CAD build for the part. Positions are in the model's coordinates, mm. A direction names the side the tool comes from. Round coordinates to 2 decimals unless told otherwise and drop trailing zeros. Write each loop counter-clockwise with the first axis right and the second up, starting at its lowest first coordinate (ties: lowest second). Pieces come first, ordered by that corner, then holes. Notation, with made-up numbers: (37.5, 69) -> (92.5, 69) arc R27 cw to (92.5, 105) -> close; hole circle Ø5 at (8.5, 34). An arc over 180 degrees is marked (long way). Answer in a Markdown table with one row per item. Add a question column.
```python
from build123d import *

# Parameters (mm, degrees)
BOSS_EXTRUDE1_DEPTH     = 56
CUT_EXTRUDE1_DEPTH      = 11
SKETCH6_R               = 11.25
SKETCH6_R_2             = 11
CUT_EXTRUDE3_DEPTH      = 7
CUT_EXTRUDE4_REACH      = 182.499
SKETCH7_R               = 1.55
SKETCH8_R               = 2.75
SKETCH8_R_2             = 1.55
CUT_EXTRUDE5_DEPTH      = 3
SKETCH9_R               = 4.5
SKETCH9_R_2             = 2.75
CUT_EXTRUDE6_DEPTH      = 5
CUT_EXTRUDE7_DEPTH      = 181.499307478
CUT_EXTRUDE7_DEPTH_BACK = 181.499307478
SKETCH9_3_R             = 2.75
FILLET1_R               = 10
FILLET2_R               = 25
FILLET3_R               = 5
FILLET4_R               = 2


with BuildPart() as part:
    # Sketch1 → Boss-Extrude1 (new, symmetric)
    with BuildSketch(Plane.XY):
        Polygon((130, 0), (130, 130), (112, 130), (112, 18), (0, 18), (0, 0), align=None)
    extrude(amount=BOSS_EXTRUDE1_DEPTH, both=True)

    # Sketch2 → Cut-Extrude1 (cut)
    with BuildSketch(Plane(origin=(130, 0, 0), x_dir=(0, 0, -1), z_dir=(1, 0, 0))):
        with BuildLine():
            Line((-20.060660172, 81.717766953), (-17.432233047, 79.089339828))
            ThreePointArc((-17.432233047, 79.089339828), (-16.945598024, 78.764180701), (-16.371572875, 78.65))
            Line((-16.371572875, 78.65), (16.371572875, 78.65))
            ThreePointArc((16.371572875, 78.65), (16.945598024, 78.764180701), (17.432233047, 79.089339828))
            Line((17.432233047, 79.089339828), (20.060660172, 81.717766953))
            ThreePointArc((20.060660172, 81.717766953), (20.385819299, 82.204401976), (20.5, 82.778427125))
            Line((20.5, 82.778427125), (20.5, 115.521572875))
            ThreePointArc((20.5, 115.521572875), (20.385819299, 116.095598024), (20.060660172, 116.582233047))
            Line((20.060660172, 116.582233047), (17.432233047, 119.210660172))
            ThreePointArc((17.432233047, 119.210660172), (16.945598024, 119.535819299), (16.371572875, 119.65))
            Line((16.371572875, 119.65), (-16.371572875, 119.65))
            ThreePointArc((-16.371572875, 119.65), (-16.945598024, 119.535819299), (-17.432233047, 119.210660172))
            Line((-17.432233047, 119.210660172), (-20.060660172, 116.582233047))
            ThreePointArc((-20.060660172, 116.582233047), (-20.385819299, 116.095598024), (-20.5, 115.521572875))
            Line((-20.5, 115.521572875), (-20.5, 82.778427125))
            ThreePointArc((-20.5, 82.778427125), (-20.385819299, 82.204401976), (-20.060660172, 81.717766953))
        make_face()
        with BuildLine():
            Line((-20.767766953, 81.010660172), (-18.139339828, 78.382233047))
            ThreePointArc((-18.139339828, 78.382233047), (-17.328281456, 77.840301169), (-16.371572875, 77.65))
            Line((-16.371572875, 77.65), (16.371572875, 77.65))
            ThreePointArc((16.371572875, 77.65), (17.328281456, 77.840301169), (18.139339828, 78.382233047))
            Line((18.139339828, 78.382233047), (20.767766953, 81.010660172))
            ThreePointArc((20.767766953, 81.010660172), (21.309698831, 81.821718544), (21.5, 82.778427125))
            Line((21.5, 82.778427125), (21.5, 115.521572875))
            ThreePointArc((21.5, 115.521572875), (21.309698831, 116.478281456), (20.767766953, 117.289339828))
            Line((20.767766953, 117.289339828), (18.139339828, 119.917766953))
            ThreePointArc((18.139339828, 119.917766953), (17.328281456, 120.459698831), (16.371572875, 120.65))
            Line((16.371572875, 120.65), (-16.371572875, 120.65))
            ThreePointArc((-16.371572875, 120.65), (-17.328281456, 120.459698831), (-18.139339828, 119.917766953))
            Line((-18.139339828, 119.917766953), (-20.767766953, 117.289339828))
            ThreePointArc((-20.767766953, 117.289339828), (-21.309698831, 116.478281456), (-21.5, 115.521572875))
            Line((-21.5, 115.521572875), (-21.5, 82.778427125))
            ThreePointArc((-21.5, 82.778427125), (-21.309698831, 81.821718544), (-20.767766953, 81.010660172))
        make_face()
    extrude(amount=-CUT_EXTRUDE1_DEPTH, mode=Mode.SUBTRACT)

    # Sketch6 → Cut-Extrude3 (cut)
    with BuildSketch(Plane.ZY.offset(-119)):
        with Locations(Location((0, 99.15, 0), (0, 0, 90))):
            Circle(SKETCH6_R)
        with Locations((0, 99.15)):
            Circle(SKETCH6_R_2, mode=Mode.SUBTRACT)
    extrude(amount=CUT_EXTRUDE3_DEPTH, mode=Mode.SUBTRACT)


with BuildPart() as cut_extrude3_kept_piece:
    # of the separate pieces the step leaves, the one the design keeps (cut_extrude3_pieces_kept)
    add(part.part.solids().sort_by_distance((130, 0, -56))[0])

    # Sketch7 → Cut-Extrude4 (cut, up to next)
    with BuildSketch(Plane.ZY.offset(-112), mode=Mode.PRIVATE) as cut_extrude4_sk1:
        with Locations(Location((-15.5, 83.65, 0), (0, 0, 270))):
            Circle(SKETCH7_R)
    cut_extrude4_tool1 = extrude(cut_extrude4_sk1.sketch, amount=-CUT_EXTRUDE4_REACH, mode=Mode.PRIVATE) & cut_extrude3_kept_piece.part
    # Sketch7 → Cut-Extrude4 (cut, up to next)
    with BuildSketch(Plane.ZY.offset(-112), mode=Mode.PRIVATE) as cut_extrude4_sk2:
        with Locations(Location((15.5, 83.65, 0), (0, 0, 270))):
            Circle(SKETCH7_R)
    cut_extrude4_tool2 = extrude(cut_extrude4_sk2.sketch, amount=-CUT_EXTRUDE4_REACH, mode=Mode.PRIVATE) & cut_extrude3_kept_piece.part
    # Sketch7 → Cut-Extrude4 (cut, up to next)
    with BuildSketch(Plane.ZY.offset(-112), mode=Mode.PRIVATE) as cut_extrude4_sk3:
        with Locations(Location((15.5, 114.65, 0), (0, 0, 270))):
            Circle(SKETCH7_R)
    cut_extrude4_tool3 = extrude(cut_extrude4_sk3.sketch, amount=-CUT_EXTRUDE4_REACH, mode=Mode.PRIVATE) & cut_extrude3_kept_piece.part
    # Sketch7 → Cut-Extrude4 (cut, up to next)
    with BuildSketch(Plane.ZY.offset(-112), mode=Mode.PRIVATE) as cut_extrude4_sk4:
        with Locations(Location((-15.5, 114.65, 0), (0, 0, 270))):
            Circle(SKETCH7_R)
    cut_extrude4_tool4 = extrude(cut_extrude4_sk4.sketch, amount=-CUT_EXTRUDE4_REACH, mode=Mode.PRIVATE) & cut_extrude3_kept_piece.part
    add(cut_extrude4_tool1.solids().sort_by_distance((112, 83.65, -15.5))[0], mode=Mode.SUBTRACT)
    add(cut_extrude4_tool2.solids().sort_by_distance((112, 83.65, 15.5))[0], mode=Mode.SUBTRACT)
    add(cut_extrude4_tool3.solids().sort_by_distance((112, 114.65, 15.5))[0], mode=Mode.SUBTRACT)
    add(cut_extrude4_tool4.solids().sort_by_distance((112, 114.65, -15.5))[0], mode=Mode.SUBTRACT)

    # Sketch8 → Cut-Extrude5 (cut)
    # profile 1 of 4: a face of its own
    with BuildSketch(Plane.ZY.offset(-112)):
        with Locations(Location((-15.5, 114.65, 0), (0, 0, 270))):
            Circle(SKETCH8_R)
        with Locations(Location((-15.5, 114.65, 0), (0, 0, 270))):
            Circle(SKETCH8_R_2, mode=Mode.SUBTRACT)
    # profile 2 of 4: a face of its own
    with BuildSketch(Plane.ZY.offset(-112)):
        with Locations(Location((15.5, 114.65, 0), (0, 0, 270))):
            Circle(SKETCH8_R)
        with Locations(Location((15.5, 114.65, 0), (0, 0, 270))):
            Circle(SKETCH8_R_2, mode=Mode.SUBTRACT)
    # profile 3 of 4: a face of its own
    with BuildSketch(Plane.ZY.offset(-112)):
        with Locations(Location((15.5, 83.65, 0), (0, 0, 270))):
            Circle(SKETCH8_R)
        with Locations(Location((15.5, 83.65, 0), (0, 0, 270))):
            Circle(SKETCH8_R_2, mode=Mode.SUBTRACT)
    # profile 4 of 4: a face of its own
    with BuildSketch(Plane.ZY.offset(-112)):
        with Locations(Location((-15.5, 83.65, 0), (0, 0, 270))):
            Circle(SKETCH8_R)
        with Locations(Location((-15.5, 83.65, 0), (0, 0, 270))):
            Circle(SKETCH8_R_2, mode=Mode.SUBTRACT)
    extrude(amount=-CUT_EXTRUDE5_DEPTH, mode=Mode.SUBTRACT)

    # Sketch9 → Cut-Extrude6 (cut)
    # profile 1 of 8: a face of its own
    with BuildSketch(Plane(origin=(0, 18, 0), x_dir=(1, 0, 0), z_dir=(0, 1, 0))):
        with Locations(Location((15, -41, 0), (0, 0, 180))):
            Circle(SKETCH9_R)
        with Locations((15, -41)):
            Circle(SKETCH9_R_2, mode=Mode.SUBTRACT)
    # profile 2 of 8: a face of its own
    with BuildSketch(Plane(origin=(0, 18, 0), x_dir=(1, 0, 0), z_dir=(0, 1, 0))):
        with Locations((15, -41)):
            Circle(SKETCH9_R_2)
    # profile 3 of 8: a face of its own
    with BuildSketch(Plane(origin=(0, 18, 0), x_dir=(1, 0, 0), z_dir=(0, 1, 0))):
        with Locations(Location((15, 41, 0), (0, 0, 180))):
            Circle(SKETCH9_R)
        with Locations((15, 41)):
            Circle(SKETCH9_R_2, mode=Mode.SUBTRACT)
    # profile 4 of 8: a face of its own
    with BuildSketch(Plane(origin=(0, 18, 0), x_dir=(1, 0, 0), z_dir=(0, 1, 0))):
        with Locations((15, 41)):
            Circle(SKETCH9_R_2)
    # profile 5 of 8: a face of its own
    with BuildSketch(Plane(origin=(0, 18, 0), x_dir=(1, 0, 0), z_dir=(0, 1, 0))):
        with Locations(Location((97, 41, 0), (0, 0, 180))):
            Circle(SKETCH9_R)
        with Locations((97, 41)):
            Circle(SKETCH9_R_2, mode=Mode.SUBTRACT)
    # profile 6 of 8: a face of its own
    with BuildSketch(Plane(origin=(0, 18, 0), x_dir=(1, 0, 0), z_dir=(0, 1, 0))):
        with Locations((97, 41)):
            Circle(SKETCH9_R_2)
    # profile 7 of 8: a face of its own
    with BuildSketch(Plane(origin=(0, 18, 0), x_dir=(1, 0, 0), z_dir=(0, 1, 0))):
        with Locations(Location((97, -41, 0), (0, 0, 180))):
            Circle(SKETCH9_R)
        with Locations((97, -41)):
            Circle(SKETCH9_R_2, mode=Mode.SUBTRACT)
    # profile 8 of 8: a face of its own
    with BuildSketch(Plane(origin=(0, 18, 0), x_dir=(1, 0, 0), z_dir=(0, 1, 0))):
        with Locations((97, -41)):
            Circle(SKETCH9_R_2)
    extrude(amount=-CUT_EXTRUDE6_DEPTH, mode=Mode.SUBTRACT)

    # Sketch9<3> → Cut-Extrude7 (cut, two sides: drawn at the far end of the back side and taken through both)
    with BuildSketch(Plane(origin=(0, 18, 0), x_dir=(1, 0, 0), z_dir=(0, 1, 0)).offset(-CUT_EXTRUDE7_DEPTH_BACK)):
        with Locations(Location((15, 41, 0), (0, 0, 180))):
            Circle(SKETCH9_3_R)
        with Locations(Location((97, 41, 0), (0, 0, 180))):
            Circle(SKETCH9_3_R)
        with Locations(Location((97, -41, 0), (0, 0, 180))):
            Circle(SKETCH9_3_R)
        with Locations(Location((15, -41, 0), (0, 0, 180))):
            Circle(SKETCH9_3_R)
    extrude(amount=CUT_EXTRUDE7_DEPTH + CUT_EXTRUDE7_DEPTH_BACK, mode=Mode.SUBTRACT)

    # Fillet1
    fillet1_edges = [cut_extrude3_kept_piece.edges().sort_by_distance(p)[0] for p in [
        (112, 18, 0),
    ]]
    fillet(fillet1_edges, radius=FILLET1_R)

    # Fillet2
    fillet2_edges = [cut_extrude3_kept_piece.edges().sort_by_distance(p)[0] for p in [
        (121, 130, -56),
        (121, 130, 56),
    ]]
    fillet(fillet2_edges, radius=FILLET2_R)

    # Fillet3
    fillet3_edges = [cut_extrude3_kept_piece.edges().sort_by_distance(p)[0] for p in [
        (130, 0, 0),
    ]]
    fillet(fillet3_edges, radius=FILLET3_R)

    # Fillet4
    fillet4_edges = [cut_extrude3_kept_piece.edges().sort_by_distance(p)[0] for p in [
        (51, 18, -56),
        (51, 18, 56),
        (109.071067812, 20.928932188, -56),
        (109.071067812, 20.928932188, 56),
        (112, 130, 0),
        (130, 130, 0),
        (112, 66.5, -56),
        (112, 66.5, 56),
        (112, 122.67766953, 48.67766953),
        (112, 122.67766953, -48.67766953),
        (130, 122.67766953, 48.67766953),
        (130, 122.67766953, -48.67766953),
        (130, 55, -56),
        (130, 55, 56),
        (128.535533906, 1.464466094, -56),
        (128.535533906, 1.464466094, 56),
        (0, 18, 0),
        (62.5, 0, -56),
        (0, 0, 0),
        (62.5, 0, 56),
        (130, 79.696446609, 19.453553391),
        (130, 81.821718544, 21.309698831),
        (130, 99.15, 21.5),
        (130, 116.478281456, 21.309698831),
        (130, 118.603553391, 19.453553391),
        (130, 120.459698831, 17.328281456),
        (130, 120.65, 0),
        (130, 120.459698831, -17.328281456),
        (130, 118.603553391, -19.453553391),
        (130, 116.478281456, -21.309698831),
        (130, 99.15, -21.5),
        (130, 81.821718544, -21.309698831),
        (130, 79.696446609, -19.453553391),
        (130, 77.840301169, -17.328281456),
        (130, 77.65, 0),
        (130, 77.840301169, 17.328281456),
    ]]
    fillet(fillet4_edges, radius=FILLET4_R)


solid = cut_extrude3_kept_piece.part
```
Item 1: Drill centre lines: probe 1 along X at (y, z) = (9, 41); probe 2 along Z at (x, y) = (15, 8); probe 3 along Z at (x, y) = (117.15, 83.65). Where is each one in solid material? Low to high.
Item 2: Saw through at D-D on z = 41. Count the separate pieces of the cut face and the enclosed holes in it, then the cut area to 3 significant figures.
Item 3: Tool access for faces 4 (the flat face through (87.4, 15.6, -56)), 5 (the flat face through (115, 113, 14)), 6 (the flat face through (97, 13, -44)), 7 (the flat face through (87.4, 15.6, 56)), 8 (the flat face through (119, 90, -9)): list every direction of +Z, -Z, +X, -X, +Y, -Y with a clear straight run to the whole face (end or side of a thin tool).
Item 4: Saw through at A-A on x = 15. Give the cut face in (y, z), then the cut area to 3 significant figures.
Item 5: Two-plate mould, pull along X, no slides. Class faces 1 (the cylindrical face through (99.747, 6.409, 41.121)), 2 (the flat face through (115, 82, 14)), 3 (the flat face through (124, 99, -21.5)): +X half, -X half, draft (parallel to the pull), parting line (faces both ways), or undercut.
Item 6: Saw through at B-B on z = -6. Give the cut face in (x, y), then the cut area to 3 significant figures.
Item 7: Saw through at C-C on x = 47. Give the cut face in (y, z), then the cut area to 3 significant figures.
Item 8: Pin check, flat tips, straight feed: pin 1 (4.5 mm diameter, centred on x = 13.5, z = -40, fed in from +Y); pin 2 (3 mm diameter, centred on y = 47.5, z = -32, fed in from -X); pin 3 (14.5 mm diameter, centred on x = 97, z = 41, fed in from +Y). Stop position of each tip, or through.
Recorded:
| question | item | result |
|---|---|---|
| 1 | probe 1 | 0 to 12.25, 17.75 to 94.25, 99.75 to 130 |
| 1 | probe 2 | -56 to -43.75, -38.25 to 38.25, 43.75 to 56 |
| 1 | probe 3 | -56 to -17.05, -13.95 to 13.95, 17.05 to 56 |
| 2 | separate pieces | 3 |
| 2 | enclosed holes | 0 |
| 2 | area | 4,100 mm2 |
| 3 | face 4 | -Z, +X, -X, +Y, -Y |
| 3 | face 5 | -X |
| 3 | face 6 | +Y |
| 3 | face 7 | +Z, +X, -X, +Y, -Y |
| 3 | face 8 | +X |
| 4 | outline | (0, -54) arc R2 ccw to (2, -56) -> (16, -56) arc R2 ccw to (18, -54) -> (18, -45.5) -> (13, -45.5) -> (13, -43.75) -> (0, -43.75) -> close; (0, -38.25) -> (13, -38.25) -> (13, -36.5) -> (18, -36.5) -> (18, 36.5) -> (13, 36.5) -> (13, 38.25) -> (0, 38.25) -> close; (0, 43.75) -> (13, 43.75) -> (13, 45.5) -> (18, 45.5) -> (18, 54) arc R2 ccw to (16, 56) -> (2, 56) arc R2 ccw to (0, 54) -> close |
| 4 | area | 1,780 mm2 |
| 5 | face 1 | undercut |
| 5 | face 2 | -X half |
| 5 | face 3 | draft |
| 6 | outline | (0, 2) arc R2 ccw to (2, 0) -> (125, 0) arc R5 ccw to (130, 5) -> (130, 75.65) arc R2 ccw to (128, 77.65) -> (119, 77.65) -> (119, 89.63) -> (112, 89.63) -> (112, 28) arc R10 cw to (102, 18) -> (2, 18) arc R2 ccw to (0, 16) -> close; (112, 108.67) -> (119, 108.67) -> (119, 120.65) -> (128, 120.65) arc R2 ccw to (130, 122.65) -> (130, 128) arc R2 ccw to (128, 130) -> (114, 130) arc R2 ccw to (112, 128) -> close |
| 6 | area | 3,760 mm2 |
| 7 | outline | (0, -54) arc R2 ccw to (2, -56) -> (16, -56) arc R2 ccw to (18, -54) -> (18, 54) arc R2 ccw to (16, 56) -> (2, 56) arc R2 ccw to (0, 54) -> close |
| 7 | area | 2,010 mm2 |
| 8 | pin 1 | y = 13 |
| 8 | pin 2 | x = 112 |
| 8 | pin 3 | y = 18.26 |
